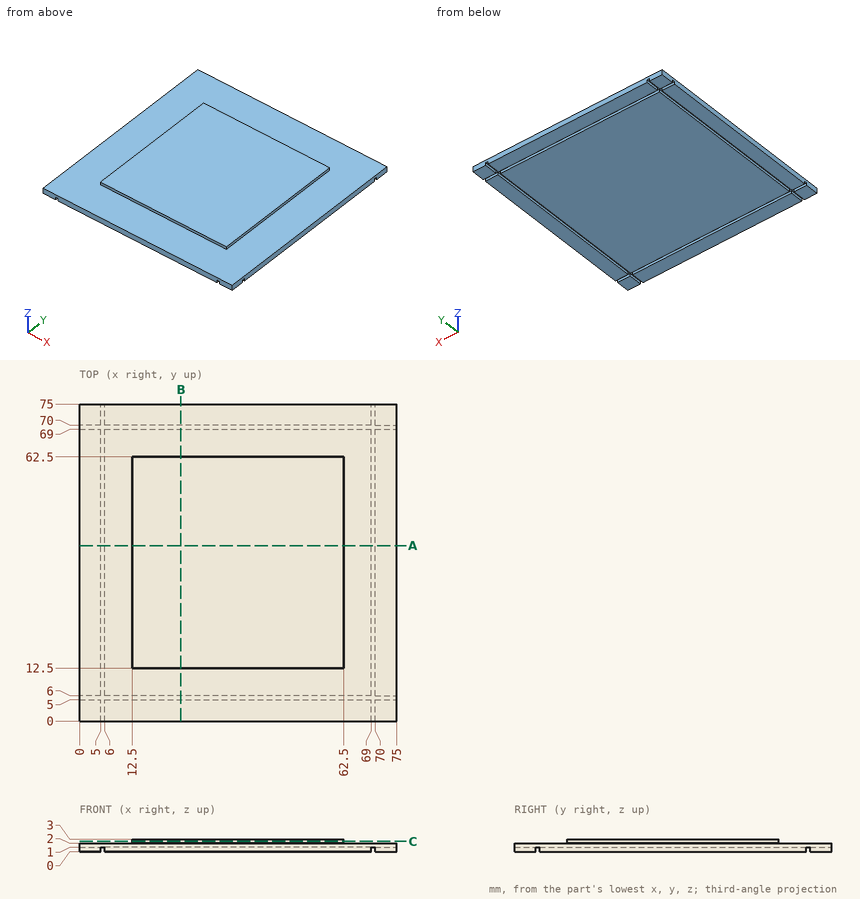
Source: three-view drawing plus pictorial views. Frame: mm from the lowest corner of the part. Give positions to 0.01 mm unless a question says otherwise; leave off trailing zeros. Order: outer loops, then holes, each group sorted by start corner. A loop starts at its lowest first (then second) coordinate and runs counter-clockwise, first axis right, second up. Notation, with made-up numbers: (57.25, 17.25) -> (104.25, 17.25) arc R25 ccw to (104.25, 37.25) -> close; hole circle Ø7 at (22, -32). An arc over 180 degrees is marked (long way). Use a Markdown table: item, result.
Q1. Section C-C (z = 2.45). Return the cut outline in (x, y).
A:
| item | result |
|---|---|
| outline | (12.5, 12.5) -> (62.5, 12.5) -> (62.5, 62.5) -> (12.5, 62.5) -> close |
Q2. Material intervals for line 1 (X direction, y = 47.5, z = 0.9); line 2 (Y direction, x = 32.5, z = 2.9), sorted ascending. Write a range as [from, to].
A:
| item | result |
|---|---|
| line 1 | [0, 5], [6, 69], [70, 75] |
| line 2 | [12.5, 62.5] |
Q3. Section A-A (y = 41.5). Return the cut outline in (x, z), and give its area (3 significant figures).
A:
| item | result |
|---|---|
| outline | (0, 0) -> (5, 0) -> (5, 1) -> (6, 1) -> (6, 0) -> (69, 0) -> (69, 1) -> (70, 1) -> (70, 0) -> (75, 0) -> (75, 2) -> (62.5, 2) -> (62.5, 3) -> (12.5, 3) -> (12.5, 2) -> (0, 2) -> close |
| area | 198 mm^2 |
Q4. First-contact query: P1, Ø0.5, axis at x = 35.5, z = 2.5, coming from the -Y side; P2, Ø0.5, axis at y = 39, z = 2.5, coming from the +X side. Flat tips, straight axial feed; report the tip coordinate or a pass-through.
A:
| item | result |
|---|---|
| P1 | y = 12.5 |
| P2 | x = 62.5 |
